Design review of the part built by this model. Coordinates are the model's own, in mm. Give positions to 0.01 mm unless a question says otherwise; leave off trailing zeros. Write each loop counter-clockwise with the first axis right and the second up, starting at its lowest first coordinate (ties: lowest second). Pieces come first, ordered by that corner, then holes.
```python
from build123d import *

# Parameters (mm, degrees)
F0_R     = 3.81
F0_R_2   = 1.3
F1_DEPTH = 5.588


with BuildPart() as f1:
    # F0 (on Top) → F1 (new body)
    with BuildSketch(Plane.XY):
        Polygon((41.4213562373, 100), (-41.4213562373, 100), (-100, 41.4213562373), (-100, -41.4213562373), (-41.4213562373, -100), (41.4213562373, -100), (100, -41.4213562373), (100, 41.4213562373), align=None)
        with Locations((-66.675, -42.85)):
            Circle(F0_R, mode=Mode.SUBTRACT)
        with Locations((-31.7881, -31.7881)):
            Circle(F0_R_2, mode=Mode.SUBTRACT)
        with Locations((31.7881, -31.7881)):
            Circle(F0_R_2, mode=Mode.SUBTRACT)
        with BuildLine():
            ThreePointArc((70.485, -42.85), (66.675, -46.66), (62.865, -42.85))
            ThreePointArc((62.865, -42.85), (66.675, -39.04), (70.485, -42.85))
        make_face(mode=Mode.SUBTRACT)
        with Locations((-31.7881, 31.7881)):
            Circle(F0_R_2, mode=Mode.SUBTRACT)
        with Locations((31.7881, 31.7881)):
            Circle(F0_R_2, mode=Mode.SUBTRACT)
    extrude(amount=F1_DEPTH)


solid = f1.part
```
(1) To check wall thickness, follow L1, parallel to Y at x = -68.5, z = 0.75; L2, parallel to Y at x = -70, z = 0.8; L3, parallel to X at y = -71, z = 4.1. State the ranges of each line that lie inside material, in increasing order.
Resolved:
L1: y = -72.92 to -46.19, -39.51 to 72.92
L2: y = -71.42 to -44.71, -40.99 to 71.42
L3: x = -70.42 to 70.42
(2) Consider section A-A, the plane z = 2.45. Give the boundary of the cut face in (x, y) (3 decimals), then the cut area to 3 significant figures.
Resolved:
outline: (-100, -41.421) - (-41.421, -100) - (41.421, -100) - (100, -41.421) - (100, 41.421) - (41.421, 100) - (-41.421, 100) - (-100, 41.421) - close; hole circle Ø7.62 at (-66.675, -42.85); hole circle Ø2.6 at (-31.788, -31.788); hole circle Ø2.6 at (-31.788, 31.788); hole circle Ø2.6 at (31.788, -31.788); hole circle Ø2.6 at (31.788, 31.788); hole circle Ø7.62 at (66.675, -42.85)
area: 33,000 mm2
(3) Clearance check with flat-ended pins moving along their axes: P1, Ø2.5, axis at x = 31.79, y = -31.79, coming from the +Z side; P2, Ø1, axis at x = 2.5, y = 14.5, coming from the -Z side. State where each tip first meets the part, or that it passes through.
Resolved:
P1: passes through
P2: stops at z = 0
(4) Mouldability with a two-part tool opening along X and no side actions: class faces 1 (the face through (100, -1, 3)), 2 (the face through (-1, 1, 0)), 3 (the face through (-64.627, -39.637, 2.755)) as pulls with the +X half, pulls with the -X half, needs draft (parallel to the pull), parting line crosses it, or undercut.
Resolved:
face 1: pulls with the +X half
face 2: needs draft
face 3: undercut
(5) Consider section B-B, the plane y = -62.5. Give the boundary of the cut face in (x, z), then the cut area to 3 significant figures.
Resolved:
outline: (-78.92, 0) - (78.92, 0) - (78.92, 5.59) - (-78.92, 5.59) - close
area: 882 mm2
